from build123d import *

# Parameters (mm, degrees)
SKETCH2_R             = 10
BOSS_EXTRUDE1_DEPTH   = 2
SKETCH3_R             = 4
BOSS_EXTRUDE2_DEPTH   = 3.6
M3X0_5_TAPPED_HOLE1_D = 2.5
SKETCH6_R             = 2.585
CUT_EXTRUDE1_DEPTH    = 3.6
SKETCH7_R             = 1.5
CUT_EXTRUDE2_DEPTH    = 3
FILLET1_R             = 0.2
CUT_EXTRUDE6_DEPTH    = 3.6
CIRPATTERN1_COUNT     = 25
CHAMFER1_SIZE         = 0.5


with BuildPart() as part:
    # Sketch2 → Boss-Extrude1 (new body)
    with BuildSketch(Plane(origin=(0, 0, 0), x_dir=(1, 0, 0), z_dir=(0, 1, 0))):
        Circle(SKETCH2_R)
    extrude(amount=BOSS_EXTRUDE1_DEPTH)

    # Sketch3 → Boss-Extrude2 (add)
    with BuildSketch(Plane(origin=(0, 2, 0), x_dir=(1, 0, 0), z_dir=(0, 1, 0))):
        Circle(SKETCH3_R)
    extrude(amount=BOSS_EXTRUDE2_DEPTH)

    # M3x0.5 Tapped Hole1 (through all)
    with Locations(Plane(origin=(0, 2, 0), x_dir=(1, 0, 0), z_dir=(0, 1, 0))):
        with Locations((0, 7), (-7, 0), (0, -7), (7, 0)):
            Hole(M3X0_5_TAPPED_HOLE1_D / 2)

    # Sketch6 → Cut-Extrude1 (cut)
    with BuildSketch(Plane(origin=(0, 5.6, 0), x_dir=(1, 0, 0), z_dir=(0, 1, 0))):
        Circle(SKETCH6_R)
    extrude(amount=-CUT_EXTRUDE1_DEPTH, mode=Mode.SUBTRACT)

    # Sketch7 → Cut-Extrude2 (cut, through all)
    with BuildSketch(Plane(origin=(0, 2, 0), x_dir=(1, 0, 0), z_dir=(0, 1, 0))):
        Circle(SKETCH7_R)
    extrude(amount=-CUT_EXTRUDE2_DEPTH, mode=Mode.SUBTRACT)

    # Fillet1
    fillet1_edges = [part.edges().sort_by_distance(p)[0] for p in [
        (-10, 0, 0),
        (-10, 2, 0),
        (-4, 2, 0),
        (-4, 5.6, 0),
    ]]
    fillet(fillet1_edges, radius=FILLET1_R)

    # Sketch8 → Cut-Extrude6 (cut)
    with BuildSketch(Plane(origin=(0, 5.6, 0), x_dir=(1, 0, 0), z_dir=(0, 1, 0))):
        with BuildLine():
            Line((2.564616503, 0.323986409), (2.89, 0))
            Line((2.89, 0), (2.564616503, -0.323986409))
            ThreePointArc((2.564616503, -0.323986409), (2.585, 0), (2.564616503, 0.323986409))
        make_face()
    cut_extrude6 = extrude(amount=-CUT_EXTRUDE6_DEPTH, mode=Mode.SUBTRACT)

    # CirPattern1: Cut-Extrude6 ×25 about axis
    cirpattern1_axis = Axis((0, 0, 0), (0, 1, 0))
    for i in range(1, CIRPATTERN1_COUNT):
        add(cut_extrude6.rotate(cirpattern1_axis, i * 360 / CIRPATTERN1_COUNT), mode=Mode.SUBTRACT)

    # Chamfer1
    chamfer1_edges = [part.edges().sort_by_distance(p)[0] for p in [
        (-1.5, 0, 0),
    ]]
    chamfer(chamfer1_edges, length=CHAMFER1_SIZE)


solid = part.part
Input: part model. Units: mm. Frame: model coordinates. A direction names the side the tool comes from. Give positions to 0.01 mm unless a question says otherwise; leave off trailing zeros. Loops run counter-clockwise (first coordinate to the right, second up) from the corner with the lowest first, then second, coordinate; pieces in that order, holes last. Notation, with made-up numbers: M -33.75,30.25 L 9.25,30.25 A32 cw 9.25,67.25 Z; hole C -5.75,-30 d2. An arc over 180 degrees is marked long. Use CSV: the item, a comma, the result in double quotes.
(1) Set-up query: faces 1 (the face through (1.3, 2, 1.2)), 2 (the face through (-0.1, 0, -2.3)). Return all of +Z, -Z, +X, -X, +Y, -Y with unobstructed straight access to the full face (end or side cutting, diameter ignored); none if empty.
Outcome:
face 1,"+Y"
face 2,"+Z, -Z, +X, -X, -Y"
(2) Material intervals for L1, parallel to Z at x = 0, y = 0.7; L2, parallel to Y at x = -3, z = 4.5; L3, parallel to X at y = 1.25, z = -7, sorted ascending. Write a range as [from, to].
Outcome:
L1,"z = [-10, -8.25], [-5.75, -1.5], [1.5, 5.75], [8.25, 10]"
L2,"y = [0, 2]"
L3,"x = [-7.14, -1.25], [1.25, 7.14]"
(3) Pin query (flat end, axial travel): P1, Ø10, axis at x = 6, z = 8, coming from the +Y side. Return the tip coordinate at first contact, or that it passes through.
Outcome:
P1,"stops at y = 2"
(4) Pull-direction query (Z, two-part tool) for faces 3 (the face through (-2.17, 0.99, 9.76)), 4 (the face through (4, 2, 2)), 5 (the face through (-5.75, 0.99, -0.05)); classes: pulls with the +Z half, pulls with the -Z half, needs draft (parallel to the pull), parting line crosses it, or undercut.
Outcome:
face 3,"parting line crosses it"
face 4,"needs draft"
face 5,"undercut"
(5) Section A-A, the plane y = 1.15. Return loops of the section in (x, z).
Outcome:
outline,"C 0,0 d20; hole C -7,0 d2.5; hole C 0,0 d3; hole C 0,-7 d2.5; hole C 0,7 d2.5; hole C 7,0 d2.5"
